from build123d import *

# Parameters (mm, degrees)
SKETCH1_W           = 31.75
SKETCH1_H           = 19.05
SKETCH1_W_2         = 3.175
SKETCH1_H_2         = 3.175
SKETCH1_W_3         = 3.2004
SKETCH1_H_3         = 3.2004
SKETCH1_W_4         = 3.2258
SKETCH1_H_4         = 3.2258
SKETCH1_W_5         = 3.2512
SKETCH1_H_5         = 3.2512
SKETCH1_W_6         = 3.2766
SKETCH1_H_6         = 3.2766
SKETCH1_W_7         = 3.048
SKETCH1_H_7         = 3.048
SKETCH1_W_8         = 3.0734
SKETCH1_H_8         = 3.0734
SKETCH1_W_9         = 3.0988
SKETCH1_H_9         = 3.0988
SKETCH1_W_10        = 3.1242
SKETCH1_H_10        = 3.1242
SKETCH1_W_11        = 3.1496
SKETCH1_H_11        = 3.1496
SKETCH1_W_12        = 3.302
SKETCH1_H_12        = 3.302
SKETCH1_W_13        = 3.3274
SKETCH1_H_13        = 3.3274
SKETCH1_W_14        = 3.3528
SKETCH1_H_14        = 3.3528
SKETCH1_W_15        = 3.3782
SKETCH1_H_15        = 3.3782
SKETCH1_W_16        = 3.4036
SKETCH1_H_16        = 3.4036
BOSS_EXTRUDE1_DEPTH = 2.54
CHAMFER1_SIZE       = 1.27
CHAMFER2_SIZE       = 0.396875


with BuildPart() as part:
    # Sketch1 → Boss-Extrude1 (new body)
    with BuildSketch(Plane(origin=(0, 0, 0), x_dir=(1, 0, 0), z_dir=(0, 1, 0))):
        with Locations((12.7, 0)):
            Rectangle(SKETCH1_W, SKETCH1_H)
        Rectangle(SKETCH1_W_2, SKETCH1_H_2, mode=Mode.SUBTRACT)
        with Locations((6.35, 0)):
            Rectangle(SKETCH1_W_3, SKETCH1_H_3, mode=Mode.SUBTRACT)
        with Locations((12.7, 0)):
            Rectangle(SKETCH1_W_4, SKETCH1_H_4, mode=Mode.SUBTRACT)
        with Locations((19.05, 0)):
            Rectangle(SKETCH1_W_5, SKETCH1_H_5, mode=Mode.SUBTRACT)
        with Locations((25.4, 0)):
            Rectangle(SKETCH1_W_6, SKETCH1_H_6, mode=Mode.SUBTRACT)
        with Locations((0, 6.35)):
            Rectangle(SKETCH1_W_7, SKETCH1_H_7, mode=Mode.SUBTRACT)
        with Locations((6.35, 6.35)):
            Rectangle(SKETCH1_W_8, SKETCH1_H_8, mode=Mode.SUBTRACT)
        with Locations((12.7, 6.35)):
            Rectangle(SKETCH1_W_9, SKETCH1_H_9, mode=Mode.SUBTRACT)
        with Locations((19.05, 6.35)):
            Rectangle(SKETCH1_W_10, SKETCH1_H_10, mode=Mode.SUBTRACT)
        with Locations((25.4, 6.35)):
            Rectangle(SKETCH1_W_11, SKETCH1_H_11, mode=Mode.SUBTRACT)
        with Locations((0, -6.35)):
            Rectangle(SKETCH1_W_12, SKETCH1_H_12, mode=Mode.SUBTRACT)
        with Locations((6.35, -6.35)):
            Rectangle(SKETCH1_W_13, SKETCH1_H_13, mode=Mode.SUBTRACT)
        with Locations((12.7, -6.35)):
            Rectangle(SKETCH1_W_14, SKETCH1_H_14, mode=Mode.SUBTRACT)
        with Locations((19.05, -6.35)):
            Rectangle(SKETCH1_W_15, SKETCH1_H_15, mode=Mode.SUBTRACT)
        with Locations((25.4, -6.35)):
            Rectangle(SKETCH1_W_16, SKETCH1_H_16, mode=Mode.SUBTRACT)
    extrude(amount=BOSS_EXTRUDE1_DEPTH)

    # Chamfer1
    chamfer1_edges = [part.edges().sort_by_distance(p)[0] for p in [
        (-3.175, 1.27, -9.525),
    ]]
    chamfer(chamfer1_edges, length=CHAMFER1_SIZE)

    # Chamfer2
    chamfer2_edges = [part.edges().sort_by_distance(p)[0] for p in [
        (14.2494, 0, -6.35),
        (12.7, 0, -7.8994),
        (11.1506, 0, -6.35),
        (12.7, 0, -4.8006),
        (14.2494, 2.54, -6.35),
        (12.7, 2.54, -7.8994),
        (11.1506, 2.54, -6.35),
        (12.7, 2.54, -4.8006),
        (20.6121, 0, -6.35),
        (19.05, 0, -7.9121),
        (17.4879, 0, -6.35),
        (19.05, 0, -4.7879),
        (20.6121, 2.54, -6.35),
        (19.05, 2.54, -7.9121),
        (17.4879, 2.54, -6.35),
        (19.05, 2.54, -4.7879),
        (28.575, 2.54, 0),
        (26.9748, 0, -6.35),
        (25.4, 0, -7.9248),
        (23.8252, 0, -6.35),
        (25.4, 0, -4.7752),
        (26.9748, 2.54, -6.35),
        (25.4, 2.54, -7.9248),
        (23.8252, 2.54, -6.35),
        (25.4, 2.54, -4.7752),
        (1.651, 0, 6.35),
        (0, 0, 4.699),
        (-1.651, 0, 6.35),
        (0, 0, 8.001),
        (1.651, 2.54, 6.35),
        (0, 2.54, 4.699),
        (-1.651, 2.54, 6.35),
        (0, 2.54, 8.001),
        (1.5875, 0, 0),
        (0, 0, -1.5875),
        (8.0137, 0, 6.35),
        (6.35, 0, 4.6863),
        (4.6863, 0, 6.35),
        (6.35, 0, 8.0137),
        (8.0137, 2.54, 6.35),
        (6.35, 2.54, 4.6863),
        (4.6863, 2.54, 6.35),
        (6.35, 2.54, 8.0137),
        (-1.5875, 0, 0),
        (0, 0, 1.5875),
        (1.5875, 2.54, 0),
        (13.335, 2.54, -9.525),
        (14.3764, 0, 6.35),
        (12.7, 0, 4.6736),
        (0, 2.54, -1.5875),
        (11.0236, 0, 6.35),
        (12.7, 0, 8.0264),
        (14.3764, 2.54, 6.35),
        (12.7, 2.54, 4.6736),
        (11.0236, 2.54, 6.35),
        (12.7, 2.54, 8.0264),
        (-1.5875, 2.54, 0),
        (0, 2.54, 1.5875),
        (20.7391, 0, 6.35),
        (19.05, 0, 4.6609),
        (17.3609, 0, 6.35),
        (19.05, 0, 8.0391),
        (20.7391, 2.54, 6.35),
        (19.05, 2.54, 4.6609),
        (17.3609, 2.54, 6.35),
        (19.05, 2.54, 8.0391),
        (27.1018, 0, 6.35),
        (25.4, 0, 4.6482),
        (23.6982, 0, 6.35),
        (25.4, 0, 8.0518),
        (27.1018, 2.54, 6.35),
        (25.4, 2.54, 4.6482),
        (23.6982, 2.54, 6.35),
        (25.4, 2.54, 8.0518),
        (-3.175, 0, 0.635),
        (-3.175, 2.54, 0.635),
        (-2.54, 0, -8.89),
        (-2.54, 2.54, -8.89),
        (7.9502, 0, 0),
        (6.35, 0, -1.6002),
        (4.7498, 0, 0),
        (6.35, 0, 1.6002),
        (7.9502, 2.54, 0),
        (6.35, 2.54, -1.6002),
        (4.7498, 2.54, 0),
        (6.35, 2.54, 1.6002),
        (14.3129, 0, 0),
        (12.7, 0, -1.6129),
        (11.0871, 0, 0),
        (12.7, 0, 1.6129),
        (14.3129, 2.54, 0),
        (12.7, 2.54, -1.6129),
        (11.0871, 2.54, 0),
        (12.7, 2.54, 1.6129),
        (13.335, 0, -9.525),
        (28.575, 0, 0),
        (20.6756, 0, 0),
        (19.05, 0, -1.6256),
        (17.4244, 0, 0),
        (19.05, 0, 1.6256),
        (20.6756, 2.54, 0),
        (19.05, 2.54, -1.6256),
        (17.4244, 2.54, 0),
        (19.05, 2.54, 1.6256),
        (12.7, 0, 9.525),
        (27.0383, 0, 0),
        (25.4, 0, -1.6383),
        (23.7617, 0, 0),
        (25.4, 0, 1.6383),
        (27.0383, 2.54, 0),
        (25.4, 2.54, -1.6383),
        (23.7617, 2.54, 0),
        (25.4, 2.54, 1.6383),
        (1.524, 0, -6.35),
        (0, 0, -7.874),
        (-1.524, 0, -6.35),
        (0, 0, -4.826),
        (1.524, 2.54, -6.35),
        (0, 2.54, -7.874),
        (-1.524, 2.54, -6.35),
        (0, 2.54, -4.826),
        (12.7, 2.54, 9.525),
        (7.8867, 0, -6.35),
        (6.35, 0, -7.8867),
        (4.8133, 0, -6.35),
        (6.35, 0, -4.8133),
        (7.8867, 2.54, -6.35),
        (6.35, 2.54, -7.8867),
        (4.8133, 2.54, -6.35),
        (6.35, 2.54, -4.8133),
    ]]
    chamfer(chamfer2_edges, length=CHAMFER2_SIZE)


solid = part.part
Work out the finished part from the listing and answer in its coordinate system (mm). A direction names the side the tool comes from. Coordinates: 2 decimals unless noted, no trailing zeros. Answer as CSV lines item,"result". Start each with the question number.
Item 1: Section A-A on x = 25.5 is taken. Give the number of separate pieces and of enclosed holes in the cut face, and give its area (3 significant figures).
Item 2: A flat-ended cylindrical pin translates along its axis: P1, Ø1, axis at x = 4.5, z = 7, coming from the -Y side. Find the tip coordinate at first contact, or state that the pin passes through.
Item 3: A tool of negligible diameter and unlimited length cuts with its end or side. For faces 1 (the face through (20.676, 1, 0)), 2 (the face through (28.575, 1, 0)), from which of +Z, -Z, +X, -X, +Y, -Y can it reach the whole face along a straight path? Write none if from no direction.
Item 4: Consider L1, parallel to X at y = 2, z = 7.25 (3 decimals); L2, parallel to X at y = 1.5, z = -0.75 (1 decimal); L3, parallel to Z at x = 19, y = 1.25 (3 decimals). Determine where each line is inside the solid, lowest interval first.
Item 5: Determine the mould class of faces 3 (the face through (-2.53, 1.26, -8.9)), 4 (the face through (12.5, 2.54, -2.2)), 5 (the face through (25, 1, 8.052)), 6 (the face through (8.014, 1, 6)) for opening direction X: released by +X, released by -X, zero draft, split by the parting line, or undercut.
Checks:
1,separate pieces,"4"
1,enclosed holes,"0"
1,area,"22.2 mm²"
2,P1,"stops at y = 0"
3,face 1,"+Y, -Y"
3,face 2,"+Z, -Z, +X, +Y, -Y"
4,L1,"x = -3.175 to -1.651, 1.651 to 4.686, 8.014 to 11.024, 14.376 to 17.361, 20.739 to 23.698, 27.102 to 28.575"
4,L2,"x = -3.2 to -1.6, 1.6 to 4.7, 8 to 11.1, 14.3 to 17.4, 20.7 to 23.8, 27 to 28.6"
4,L3,"z = -9.525 to -7.912, -4.788 to -1.626, 1.626 to 4.661, 8.039 to 9.525"
5,face 3,"released by -X"
5,face 4,"zero draft"
5,face 5,"undercut"
5,face 6,"undercut"
